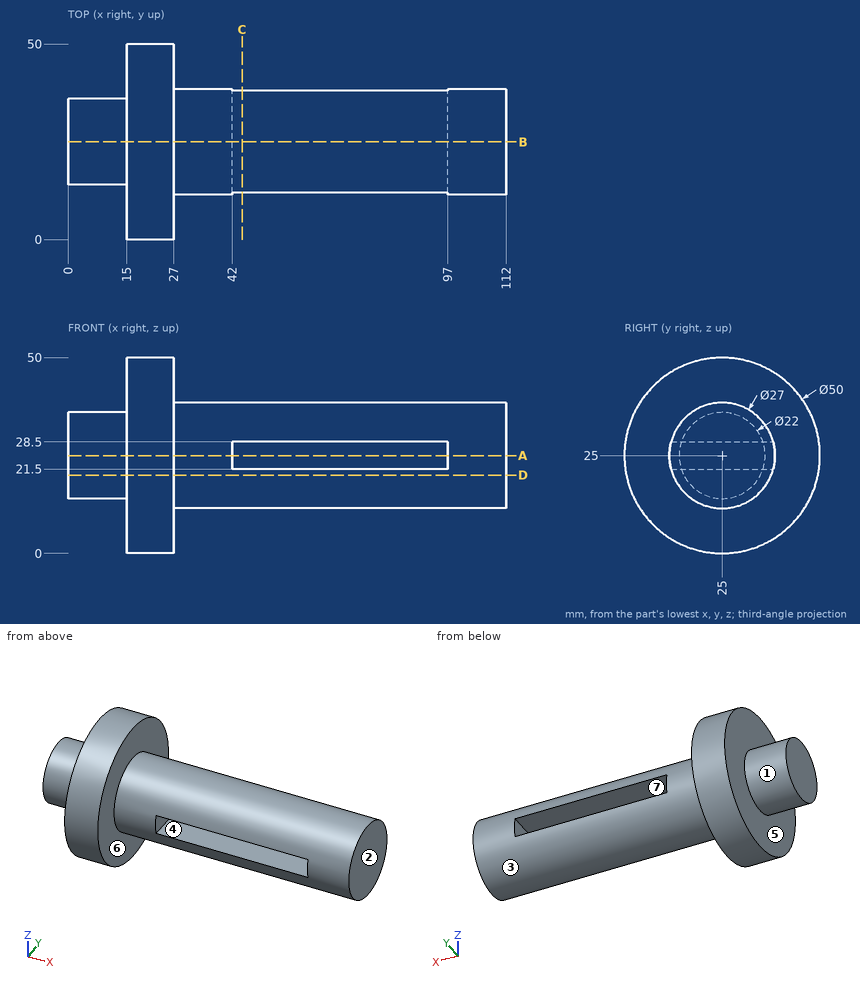
Input: dimensioned drawing with shaded views. Units: mm. Origin: part minimum x, y, z. A direction names the side the tool comes from. Coordinates: 2 decimals unless noted, no trailing zeros. Loops run counter-clockwise (first coordinate to the right, second up) from the corner with the lowest first, then second, coordinate; pieces in that order, holes last. Notation, with made-up numbers: (28.25, -12) -> (68.25, -12) arc R29 ccw to (68.25, 12) -> close; hole circle Ø10 at (54.5, -33). An arc over 180 degrees is marked (long way). One line per item, written item: value. Start each with the question number.
Q1. Contact query for flat-ended pins moving along their axis: P1, Ø6, axis at x = 22, z = 17.5, coming from the +Y side; P2, Ø3, axis at x = 48.5, y = 19.5, coming from the -Z side; P3, Ø13, axis at x = 72.5, y = 26.5, coming from the +Z side. Output: stop coordinate, or through.
Q2. Section query C-C, the plane x = 44.5. Return the cut outline in (y, z).
Q3. Section query B-B, the plane y = 25. Return the cut outline in (x, z), and give its area (3 significant figures).
Q4. Mould query, pull axis X, two halves, no side actions, for the marked faces 5, 6 and 7. Classes: pulls with the +X half, pulls with the -X half, needs draft (parallel to the pull), parting line crosses it, or undercut.
Q5. Section query D-D, the plane z = 20. Return the cut outline in (x, y).
Q6. Set-up query: the marked faces 1, 2, 3 and 4. Return all of +Z, -Z, +X, -X, +Y, -Y with unobstructed straight access to the full face (end or side cutting, diameter ignored); none if empty.
Q7. Line query: line 1 along X through (y, z) = (35, 13); line 2 along Y through (x, z) = (5.5, 25); line 3 along Y through (x, z) = (41, 31.5). Output: solid intervals per line, ascending.
Q8. Section query A-A, the plane z = 25. Return the cut outline in (x, y).
Results:
1. P1: y = 49.59
1. P2: z = 12.11
1. P3: z = 38.5
2. outline: (11.96, 21.5) arc R13.5 ccw to (38.04, 21.5) -> close; (11.96, 28.5) -> (38.04, 28.5) arc R13.5 ccw to start
3. outline: (0, 14) -> (15, 14) -> (15, 0) -> (27, 0) -> (27, 11.5) -> (112, 11.5) -> (112, 38.5) -> (27, 38.5) -> (27, 50) -> (15, 50) -> (15, 36) -> (0, 36) -> close; hole (42, 21.5) -> (97, 21.5) -> (97, 28.5) -> (42, 28.5) -> close
3. area: 2,840 mm^2
4. face 5: pulls with the -X half
4. face 6: pulls with the +X half
4. face 7: undercut
5. outline: (0, 15.2) -> (15, 15.2) -> (15, 0.51) -> (27, 0.51) -> (27, 12.46) -> (112, 12.46) -> (112, 37.54) -> (27, 37.54) -> (27, 49.49) -> (15, 49.49) -> (15, 34.8) -> (0, 34.8) -> close
6. face 1: -X
6. face 2: +Z, -Z, +X, +Y, -Y
6. face 3: +X
6. face 4: +Y, -Y
7. line 1: 15 to 27
7. line 2: 14 to 36
7. line 3: 13.17 to 36.83
8. outline: (0, 14) -> (15, 14) -> (15, 0) -> (27, 0) -> (27, 11.5) -> (42, 11.5) -> (42, 38.5) -> (27, 38.5) -> (27, 50) -> (15, 50) -> (15, 36) -> (0, 36) -> close; (97, 11.5) -> (112, 11.5) -> (112, 38.5) -> (97, 38.5) -> close
